```python
from build123d import *

# Parameters (mm, degrees)
SKETCH015_W      = 125.000379
SKETCH015_H      = 96.004006
EXTRUDE013_DEPTH = 3
SKETCH004_R      = 3.75
HOLE001_DEPTH    = 3
SKETCH005_R      = 3.25
HOLE002_DEPTH    = 3
SKETCH007_R      = 3.75
HOLE003_DEPTH    = 3
SKETCH006_R      = 1.35
HOLE004_DEPTH    = 3
SKETCH008_W      = 57.1
SKETCH008_H      = 30.66
POCKET_DEPTH     = 3
SKETCH021_R      = 1.6
HOLE007_DEPTH    = 3
HOLE007_TIPS_R   = 1.6
FILLET_R         = 2
FILLET001_R      = 2
CHAMFER_SIZE     = 1


with BuildPart() as part:
    # Sketch015 → Extrude013 (new body)
    with BuildSketch(Plane.XY):
        with Locations((15.049815, 71.702003)):
            Rectangle(SKETCH015_W, SKETCH015_H)
    extrude(amount=EXTRUDE013_DEPTH)

    # Sketch004 (on Face6 of Extrude013) → Hole001 (cut)
    with BuildSketch(Plane.XY.offset(3)):
        with Locations((-25.4, 43.200001)):
            Circle(SKETCH004_R)
    extrude(amount=-HOLE001_DEPTH, mode=Mode.SUBTRACT)

    # Sketch005 (on Face5 of Hole001) → Hole002 (cut)
    with BuildSketch(Plane.XY.offset(3)):
        with Locations((-25.299999, 87.769998)):
            Circle(SKETCH005_R)
    extrude(amount=-HOLE002_DEPTH, mode=Mode.SUBTRACT)

    # Sketch007 (on Face5 of Hole002) → Hole003 (cut)
    with BuildSketch(Plane.XY.offset(3)):
        with Locations((-6.67, 43.199999)):
            Circle(SKETCH007_R)
        with Locations((12.368629, 43.200002)):
            Circle(SKETCH007_R)
        with Locations((31.429999, 43.199999)):
            Circle(SKETCH007_R)
        with Locations((50.469999, 43.199999)):
            Circle(SKETCH007_R)
    extrude(amount=-HOLE003_DEPTH, mode=Mode.SUBTRACT)

    # Sketch006 (on Face5 of Hole003) → Hole004 (cut)
    with BuildSketch(Plane.XY.offset(3)):
        with Locations((-10.85, 65.069999)):
            Circle(SKETCH006_R)
        with Locations((54.649999, 65.069999)):
            Circle(SKETCH006_R)
        with Locations((54.649999, 108.529998)):
            Circle(SKETCH006_R)
        with Locations((-10.85, 108.519998)):
            Circle(SKETCH006_R)
    extrude(amount=-HOLE004_DEPTH, mode=Mode.SUBTRACT)

    # Sketch008 (on Face5 of Hole004) → Pocket (cut)
    with BuildSketch(Plane.XY.offset(3)):
        with Locations((22.05, 89.549998)):
            Rectangle(SKETCH008_W, SKETCH008_H)
    extrude(amount=-POCKET_DEPTH, mode=Mode.SUBTRACT)

    # Sketch021 (on Face5 of Pocket) → Hole007 (cut)
    with BuildSketch(Plane.XY.offset(3)):
        with Locations((-40.227337, 30.97648)):
            Circle(SKETCH021_R)
        with Locations((-40.231945, 70.133278)):
            Circle(SKETCH021_R)
        with Locations((-40.231026, 112.471214)):
            Circle(SKETCH021_R)
        with Locations((70.273193, 112.478386)):
            Circle(SKETCH021_R)
        with Locations((70.276276, 73.322159)):
            Circle(SKETCH021_R)
        with Locations((70.272247, 30.977751)):
            Circle(SKETCH021_R)
    extrude(amount=-HOLE007_DEPTH, mode=Mode.SUBTRACT)

    # Hole007 tips → Hole007 tip 1 section 0
    with BuildSketch(Plane.XY, mode=Mode.PRIVATE) as hole007_tip_1_s0:
        with Locations((-40.227337, 30.97648)):
            Circle(HOLE007_TIPS_R)
    loft([hole007_tip_1_s0.sketch, Vertex(-40.227337, 30.97648, -0.961377)], mode=Mode.SUBTRACT)

    # Hole007 tips → Hole007 tip 2 section 0
    with BuildSketch(Plane.XY, mode=Mode.PRIVATE) as hole007_tip_2_s0:
        with Locations((-40.231945, 70.133278)):
            Circle(HOLE007_TIPS_R)
    loft([hole007_tip_2_s0.sketch, Vertex(-40.231945, 70.133278, -0.961377)], mode=Mode.SUBTRACT)

    # Hole007 tips → Hole007 tip 3 section 0
    with BuildSketch(Plane.XY, mode=Mode.PRIVATE) as hole007_tip_3_s0:
        with Locations((-40.231026, 112.471214)):
            Circle(HOLE007_TIPS_R)
    loft([hole007_tip_3_s0.sketch, Vertex(-40.231026, 112.471214, -0.961377)], mode=Mode.SUBTRACT)

    # Hole007 tips → Hole007 tip 4 section 0
    with BuildSketch(Plane.XY, mode=Mode.PRIVATE) as hole007_tip_4_s0:
        with Locations((70.273193, 112.478386)):
            Circle(HOLE007_TIPS_R)
    loft([hole007_tip_4_s0.sketch, Vertex(70.273193, 112.478386, -0.961377)], mode=Mode.SUBTRACT)

    # Hole007 tips → Hole007 tip 5 section 0
    with BuildSketch(Plane.XY, mode=Mode.PRIVATE) as hole007_tip_5_s0:
        with Locations((70.276276, 73.322159)):
            Circle(HOLE007_TIPS_R)
    loft([hole007_tip_5_s0.sketch, Vertex(70.276276, 73.322159, -0.961377)], mode=Mode.SUBTRACT)

    # Hole007 tips → Hole007 tip 6 section 0
    with BuildSketch(Plane.XY, mode=Mode.PRIVATE) as hole007_tip_6_s0:
        with Locations((70.272247, 30.977751)):
            Circle(HOLE007_TIPS_R)
    loft([hole007_tip_6_s0.sketch, Vertex(70.272247, 30.977751, -0.961377)], mode=Mode.SUBTRACT)

    # Fillet
    fillet_edges = [part.edges().sort_by_distance(p)[0] for p in [
        (15.049814, 23.7, 3),
        (-47.450375, 23.7, 1.5),
        (-47.450375, 71.702003, 3),
        (-47.450375, 119.704006, 1.5),
        (15.049814, 119.704006, 3),
        (77.550004, 119.704006, 1.5),
        (77.550004, 71.702003, 3),
        (77.550004, 23.7, 1.5),
    ]]
    fillet(fillet_edges, radius=FILLET_R)

    # Fillet001
    fillet001_edges = [part.edges().sort_by_distance(p)[0] for p in [
        (-6.5, 89.549998, 3),
        (22.05, 104.879998, 3),
        (50.6, 89.549998, 3),
        (22.05, 74.219998, 3),
    ]]
    fillet(fillet001_edges, radius=FILLET001_R)

    # Chamfer
    chamfer_edges = [part.edges().sort_by_distance(p)[0] for p in [
        (51.307902, 105.5879, 2.526592),
        (51.307902, 73.512096, 2.526592),
        (-7.207902, 73.512096, 2.526592),
        (-7.207902, 105.5879, 2.526592),
    ]]
    chamfer(chamfer_edges, length=CHAMFER_SIZE)


with BuildPart() as part_1:
    # Body001 placement: moved
    add(part.part.moved(Location((0, 0, 24.7))))


solid = part_1.part
```
Can you work these out from the model? Positions are in its coordinate system, mm. Coordinates: 2 decimals unless noted, no trailing zeros. Loops run counter-clockwise (first coordinate to the right, second up) from the corner with the lowest first, then second, coordinate; pieces in that order, holes last. Notation, with made-up numbers: M 8,-32 L 62,-32 A19 ccw 62,-2 Z; hole C 78,76.5 d6. An arc over 180 degrees is marked long. Put each result on its own line as item: value. Start each with the question number.
(1) I need wall thicknesses on probe 1 along Y at (x, z) = (70, 25.65); probe 2 along Y at (x, z) = (10, 26.15); probe 3 along Y at (x, z) = (1, 25.85). Which ranges of each line are inside material? Lowest first, please.
(2) Imagine slicing it at D-D on z = 26.65. Give the number of separate pieces and of enclosed holes in the cut face, and give its area (3 significant figures).
(3) We'd pull the mould along X, two halves only. Please class faces 1 (the face through (54.474, 66.409, 26.221)), 2 (the face through (14, 62, 27.7)): +X half, -X half, draft (parallel to the pull), parting line (faces both ways), or undercut.
(4) Imagine slicing it at A-A on y = 65.07. List the corners of the cut face in (x, z) for me, and give its area (3 significant figures).
(5) Imagine slicing it at C-C on x = 11. List the corners of the cut face in (y, z) for me, and give its area (3 significant figures).
(6) Will this pin go through, and if not, where does the flat tip stop? pin 1 Ø3 at (x, y) = (51, 89) entering from +Z.
(7) Imagine slicing it at B-B on x = 32. List the corners of the cut face in (y, z) for me, and give its area (3 significant figures).
Worked answers:
1. probe 1: y = 23.7 to 29.4, 32.55 to 71.75, 74.9 to 110.9, 114.05 to 119.7
1. probe 2: y = 23.75 to 40.29, 46.11 to 74.17, 104.93 to 119.65
1. probe 3: y = 23.71 to 74.21, 104.89 to 119.7
2. separate pieces: 1
2. enclosed holes: 17
2. area: 9,780 mm2
3. face 1: undercut
3. face 2: draft
4. outline: M -47.45,24.7 L -12.2,24.7 L -12.2,27.7 L -45.45,27.7 A2 ccw -47.45,25.7 Z; M -9.5,24.7 L 53.3,24.7 L 53.3,27.7 L -9.5,27.7 Z; M 56,24.7 L 77.55,24.7 L 77.55,25.7 A2 ccw 75.55,27.7 L 56,27.7 Z
4. area: 357 mm2
5. outline: M 23.7,24.7 L 39.71,24.7 L 39.71,27.7 L 25.7,27.7 A2 ccw 23.7,25.7 Z; M 46.69,24.7 L 74.22,24.7 L 74.22,25.7 A2 ccw 72.22,27.7 L 46.69,27.7 Z; M 104.88,24.7 L 119.7,24.7 L 119.7,25.7 A2 ccw 117.7,27.7 L 106.88,27.7 A2 ccw 104.88,25.7 Z
5. area: 172 mm2
6. pin 1: stops at z = 27.7
7. outline: M 23.7,24.7 L 39.49,24.7 L 39.49,27.7 L 25.7,27.7 A2 ccw 23.7,25.7 Z; M 46.91,24.7 L 74.22,24.7 L 74.22,25.7 A2 ccw 72.22,27.7 L 46.91,27.7 Z; M 104.88,24.7 L 119.7,24.7 L 119.7,25.7 A2 ccw 117.7,27.7 L 106.88,27.7 A2 ccw 104.88,25.7 Z
7. area: 170 mm2
